from build123d import *

# Parameters (mm, degrees)
SKETCH1_W               = 55
SKETCH1_H               = 75
BOSS_EXTRUDE1_DEPTH     = 5
SKETCH5_W               = 5
SKETCH5_H               = 30
SKETCH5_W_2             = 15
SKETCH5_H_2             = 5
CUT_EXTRUDE3_DEPTH      = 1
CUT_EXTRUDE3_DEPTH_BACK = 6
CUT_EXTRUDE4_DEPTH      = 2.5
SKETCH7_R               = 6
CUT_EXTRUDE5_DEPTH      = 6
SKETCH8_R               = 1.59
CUT_EXTRUDE6_DEPTH      = 6


with BuildPart() as part:
    # Sketch1 → Boss-Extrude1 (new body)
    with BuildSketch(Plane(origin=(0, 0, 0), x_dir=(1, 0, 0), z_dir=(0, 1, 0))):
        with Locations((27.5, 37.5)):
            Rectangle(SKETCH1_W, SKETCH1_H)
    extrude(amount=BOSS_EXTRUDE1_DEPTH)

    # Sketch5 → Cut-Extrude3 (cut, two sides)
    with BuildSketch(Plane(origin=(0, 5, 0), x_dir=(1, 0, 0), z_dir=(0, 1, 0))) as cut_extrude3_sk:
        with Locations((2.5, 37.5)):
            Rectangle(SKETCH5_W, SKETCH5_H)
        with Locations((27.5, 72.5)):
            Rectangle(SKETCH5_W_2, SKETCH5_H_2)
        with Locations((52.5, 37.5)):
            Rectangle(SKETCH5_W, SKETCH5_H)
        with Locations((27.5, 2.5)):
            Rectangle(SKETCH5_W_2, SKETCH5_H_2)
    extrude(amount=CUT_EXTRUDE3_DEPTH, mode=Mode.SUBTRACT)
    extrude(cut_extrude3_sk.sketch, amount=-CUT_EXTRUDE3_DEPTH_BACK, mode=Mode.SUBTRACT)

    # Sketch6 → Cut-Extrude4 (cut)
    with BuildSketch(Plane.XZ):
        with BuildLine():
            Line((7.3375, -70), (47.6625, -70))
            ThreePointArc((47.6625, -70), (48.785032015, -69.535032015), (49.25, -68.4125))
            Line((49.25, -68.4125), (49.25, -28.0875))
            ThreePointArc((49.25, -28.0875), (48.785032015, -26.964967985), (47.6625, -26.5))
            Line((47.6625, -26.5), (7.3375, -26.5))
            ThreePointArc((7.3375, -26.5), (6.214967985, -26.964967985), (5.75, -28.0875))
            Line((5.75, -28.0875), (5.75, -68.4125))
            ThreePointArc((5.75, -68.4125), (6.214967985, -69.535032015), (7.3375, -70))
        make_face()
    extrude(amount=-CUT_EXTRUDE4_DEPTH, mode=Mode.SUBTRACT)

    # Sketch7 → Cut-Extrude5 (cut, through all)
    with BuildSketch(Plane(origin=(0, 5, 0), x_dir=(1, 0, 0), z_dir=(0, 1, 0))):
        with Locations((16.5, 15.75)):
            Circle(SKETCH7_R)
        with Locations((38.5, 15.75)):
            Circle(SKETCH7_R)
    extrude(amount=-CUT_EXTRUDE5_DEPTH, mode=Mode.SUBTRACT)

    # Sketch8 → Cut-Extrude6 (cut, through all)
    with BuildSketch(Plane.XZ):
        with Locations((5, -22.5)):
            Circle(SKETCH8_R)
        with Locations((20, -5)):
            Circle(SKETCH8_R)
        with Locations((35, -5)):
            Circle(SKETCH8_R)
        with Locations((50, -22.5)):
            Circle(SKETCH8_R)
        with Locations((50, -52.5)):
            Circle(SKETCH8_R)
        with Locations((35, -70)):
            Circle(SKETCH8_R)
        with Locations((20, -70)):
            Circle(SKETCH8_R)
        with Locations((5, -52.5)):
            Circle(SKETCH8_R)
    extrude(amount=-CUT_EXTRUDE6_DEPTH, mode=Mode.SUBTRACT)


solid = part.part
The listing builds one solid part. Answer for the finished solid, in the listing's coordinates (mm). A direction names the side the tool comes from. Coordinates: 2 decimals unless noted, no trailing zeros. Order: outer loops, then holes, each group sorted by start corner. A loop starts at its lowest first (then second) coordinate and runs counter-clockwise, first axis right, second up.
Q1. A cutting plane is placed at D-D, the plane x = 28. Write down the section's boundary in (y, z), and give its area (3 significant figures).
Q2. A cutting plane is placed at B-B, the plane x = 38.5. Write down the section's boundary in (y, z).
Q3. Consider line 1 (X direction, y = 1.45, z = -15.75); line 2 (X direction, y = 2.2, z = -55.5). Determine where each line is inside the solid, lowest interval first.
Q4. A cutting plane is placed at A-A, the plane y = 4.2. State how many separate pieces and enclosed holes the cut face has, and give its area (3 significant figures).
Q5. Given P1, Ø2.5, axis at x = 29.5, y = 3, coming from the +Z side; P2, Ø3, axis at x = 26.5, y = 3.5, coming from the -Z side; P3, Ø1.2, axis at y = 1, z = -45, coming from the -X side; P4, Ø3, axis at y = 1, z = -59, coming from the -X side, each flat-ended and moving along its own axis, determine where each tip first touches the part or whether it passes through.
Q6. Which of the six approach directions +Z, -Z, +X, -X, +Y, -Y give full straight-line access (tool end or side, diameter ignored) to faces 1 (the face through (20, 3, -2)), 2 (the face through (5, 3, -37)), 3 (the face through (53, 3, -52.5))?
Q7. For a pull along X with two mould halves and no side action, classify faces 4 (the face through (28, 1, -26.5)), 5 (the face through (50, 3, -37)), 6 (the face through (0, 2, -11)), 7 (the face through (27, 3, -5)) as pulls with the +X half, pulls with the -X half, needs draft (parallel to the pull), parting line crosses it, or undercut.
Q8. A cutting plane is placed at C-C, the plane z = -65.5. Write down the section's boundary in (x, y).
Answers follow:
1. outline: (0, -26.5) - (2.5, -26.5) - (2.5, -70) - (5, -70) - (5, -5) - (0, -5) - close
1. area: 216 mm2
2. outline: (0, -75) - (5, -75) - (5, -21.75) - (0, -21.75) - (0, -26.5) - (2.5, -26.5) - (2.5, -70) - (0, -70) - close; (0, -9.75) - (5, -9.75) - (5, 0) - (0, 0) - close
3. line 1: x = 0 to 10.5, 22.5 to 32.5, 44.5 to 55
3. line 2: x = 0 to 5.75, 49.25 to 55
4. separate pieces: 1
4. enclosed holes: 2
4. area: 3,400 mm2
5. P1: stops at z = -5
5. P2: stops at z = -70
5. P3: stops at x = 5
5. P4: stops at x = 0
6. face 1: +Z, +Y, -Y
6. face 2: -X, +Y, -Y
6. face 3: +X, +Y, -Y
7. face 4: undercut
7. face 5: pulls with the +X half
7. face 6: pulls with the -X half
7. face 7: undercut
8. outline: (0, 0) - (5.75, 0) - (5.75, 2.5) - (49.25, 2.5) - (49.25, 0) - (55, 0) - (55, 5) - (0, 5) - close
